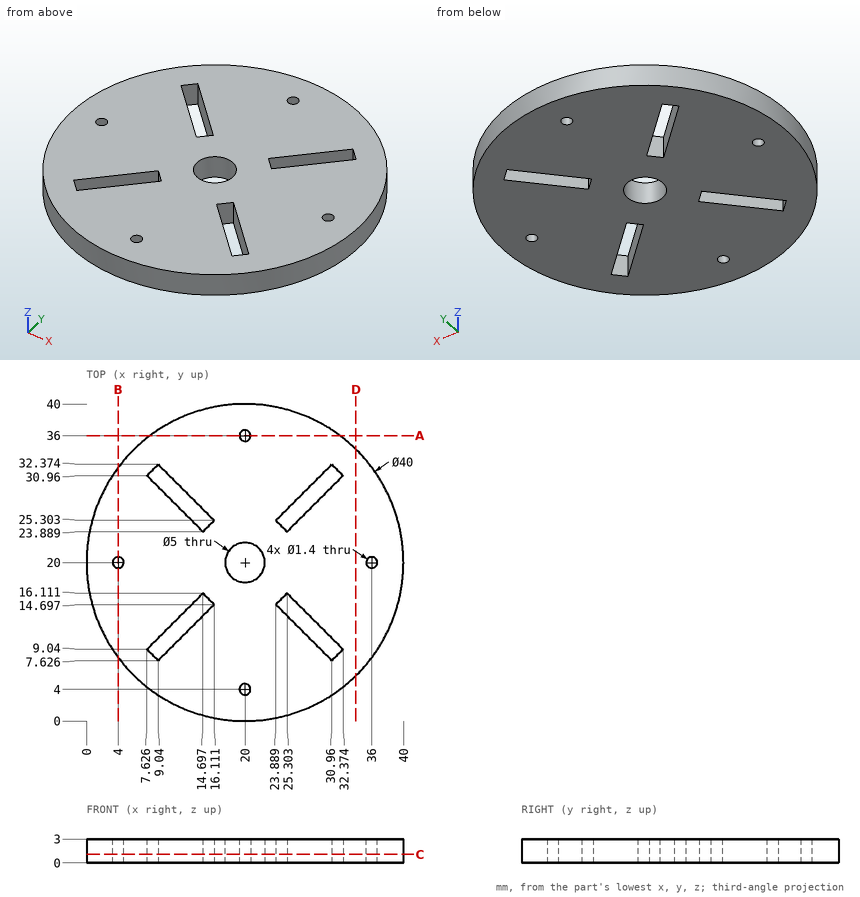
Source: three-view drawing plus pictorial views. Frame: mm from the lowest corner of the part. Round coordinates to 2 decimals unless told otherwise and drop trailing zeros. Order: outer loops, then holes, each group sorted by start corner. A loop starts at its lowest first (then second) coordinate and runs counter-clockwise, first axis right, second up. Notation, with made-up numbers: M -36,25 L -7,25 A23 ccw -7,51 Z; hole C 8,9 d10. An arc over 180 degrees is marked long. One line per item, written item: value.
(1) Cut plane D-D (x = 34). Return the cut outline in (y, z).
Result sheet:
outline: M 5.72,0 L 34.28,0 L 34.28,3 L 5.72,3 Z
(2) Cut plane C-C (z = 1.05). Give the number of separate pieces and of enclosed holes in the cut face, and give its area (3 significant figures).
Result sheet:
separate pieces: 1
enclosed holes: 9
area: 1,150 mm2
(3) Cut plane A-A (y = 36). Return the cut outline in (x, z).
Result sheet:
outline: M 8,0 L 19.3,0 L 19.3,3 L 8,3 Z; M 20.7,0 L 32,0 L 32,3 L 20.7,3 Z
(4) Line query: probe 1 along Y at (x, z) = (20, 2.2); probe 2 along Y at (x, z) = (31, 1.8) (1 decimal); probe 3 along X at (y, z) = (11, 0.65) (1 decimal). Output: solid intervals per line, ascending. Write a range as [from, to].
Result sheet:
probe 1: [0, 3.3], [4.7, 17.5], [22.5, 35.3], [36.7, 40]
probe 2: [3.3, 7.7], [10.4, 29.6], [32.3, 36.7]
probe 3: [2.1, 9.6], [12.4, 27.6], [30.4, 37.9]
(5) Pin query (flat end, axial travel): P1, Ø0.8, axis at x = 20, y = 36, coming from the -Z side (3 decimals). Return the tip coordinate at first contact, or that it passes through.
Result sheet:
P1: through
